from build123d import *

# Parameters (mm, degrees)
F0_R         = 1.745
F1_DEPTH     = 1.66
F2_R         = 4
F3_T1_DEPTH  = 11.0406372139
F3_T3_DEPTH  = 2.9562992506
F3_T5_DEPTH  = 2.7192996153
F3_T7_DEPTH  = 12.9650408158
F3_T9_DEPTH  = 2.8625815694
F3_T11_DEPTH = 2.7133982533


# Not quite as in the source:
# - a fillet or chamfer that OpenCascade refuses, or shapes differently, is made with other operations: its cross-section is extruded or revolved along the edge and cut away or added


with BuildPart() as f1:
    # F0 (on Top) → F1 (new body)
    with BuildSketch(Plane.XY):
        with BuildLine():
            Line((9.301183783, 21.0652845629), (-9.82, 21.0652845629))
            Line((-9.82, 21.0652845629), (-9.82, 16.2710778286))
            Line((-9.82, 16.2710778286), (-6.76, 13.7425599752))
            Line((-6.76, 13.7425599752), (-6.76, 6.5925599752))
            Line((-6.76, 6.5925599752), (-9.82, 4.2610778286))
            Line((-9.82, 4.2610778286), (-9.82, 0.8810778286))
            Line((-9.82, 0.8810778286), (-9.82, -30.8189221714))
            Line((-9.82, -30.8189221714), (-6.5227223381, -36.7505173139))
            Line((-6.5227223381, -36.7505173139), (-3.43, -30.6931023543))
            Line((-3.43, -30.6931023543), (-3.43, 0))
            ThreePointArc((-3.43, 0), (0, 3.43), (3.43, 0))
            Line((3.43, 0), (3.43, -30.6931023543))
            Line((3.43, -30.6931023543), (6.4156440855, -37.4231023543))
            Line((6.4156440855, -37.4231023543), (9.301183783, -30.87889562))
            Line((9.301183783, -30.87889562), (9.301183783, 1.0068976457))
            Line((9.301183783, 1.0068976457), (9.4504277734, 4.2610778286))
            Line((9.4504277734, 4.2610778286), (6.5356440855, 6.7183797924))
            Line((6.5356440855, 6.7183797924), (6.5356440855, 13.8683797924))
            Line((6.5356440855, 13.8683797924), (9.2185314492, 16.0852845629))
            Line((9.2185314492, 16.0852845629), (9.301183783, 21.0652845629))
        make_face()
        with Locations((-6.686183783, 18.82610438)):
            Circle(F0_R, mode=Mode.SUBTRACT)
        with Locations((6.686183783, 18.7002845629)):
            Circle(F0_R, mode=Mode.SUBTRACT)
    extrude(amount=F1_DEPTH)

    # F2
    f2_edges = [f1.edges().sort_by_distance(p)[0] for p in [
        (-6.76, 6.59256, 0.83),
        (-6.76, 13.74256, 0.83),
        (6.535644, 6.71838, 0.83),
        (6.535644, 13.86838, 0.83),
    ]]
    fillet(f2_edges, radius=F2_R)

    # F3: fillet of radius 1 on 6 edges, made by hand

    # F3_s2 → F3_t1 (cut)
    with BuildSketch(Plane.XY.offset(-4.690318607)):
        with BuildLine():
            add(Edge.make_bspline(
                [(-7.4342616517, -35.110715417), (-6.5227223381, -36.7505173139), (-5.6695955837, -35.0795807734)],
                knots=[0, 0, 0, 1, 1, 1], degree=2, weights=[1, 1, 1]))
            Line((-5.6695955837, -35.0795807734), (-6.5227223381, -36.7505173139))
            Line((-6.5227223381, -36.7505173139), (-7.4342616517, -35.110715417))
        make_face()
    extrude(amount=F3_T1_DEPTH, mode=Mode.SUBTRACT)

    # F3_s4 → F3_t3 (cut)
    with BuildSketch(Plane.XY.offset(-0.6481496253)):
        with BuildLine():
            add(Edge.make_bspline(
                [(-9.82, -30.5596623213), (-9.82, -30.8189221714), (-9.6940354517, -31.0455244716)],
                knots=[0, 0, 0, 1, 1, 1], degree=2, weights=[1, 1, 1]))
            Line((-9.6940354517, -31.0455244716), (-9.82, -30.8189221714))
            Line((-9.82, -30.8189221714), (-9.82, -30.5596623213))
        make_face()
    extrude(amount=F3_T3_DEPTH, mode=Mode.SUBTRACT)

    # F3_s6 → F3_t5 (cut)
    with BuildSketch(Plane.XY.offset(-0.5296498077)):
        with BuildLine():
            add(Edge.make_bspline(
                [(3.43, -30.4812424312), (3.43, -30.6931023543), (3.5159130776, -30.8867607393)],
                knots=[0, 0, 0, 1, 1, 1], degree=2, weights=[1, 1, 1]))
            Line((3.5159130776, -30.8867607393), (3.43, -30.6931023543))
            Line((3.43, -30.6931023543), (3.43, -30.4812424312))
        make_face()
    extrude(amount=F3_T5_DEPTH, mode=Mode.SUBTRACT)

    # F3_s8 → F3_t7 (cut)
    with BuildSketch(Plane.XY.offset(-5.6525204079)):
        with BuildLine():
            add(Edge.make_bspline(
                [(5.4987638806, -35.3563443608), (6.4156440855, -37.4231023543), (7.3278517341, -35.3542777798)],
                knots=[0, 0, 0, 1, 1, 1], degree=2, weights=[1, 1, 1]))
            Line((7.3278517341, -35.3542777798), (6.4156440855, -37.4231023543))
            Line((6.4156440855, -37.4231023543), (5.4987638806, -35.3563443608))
        make_face()
    extrude(amount=F3_T7_DEPTH, mode=Mode.SUBTRACT)

    # F3_s10 → F3_t9 (cut)
    with BuildSketch(Plane.XY.offset(-0.6012907847)):
        with BuildLine():
            add(Edge.make_bspline(
                [(-3.5393693837, -30.9073135471), (-3.43, -30.6931023543), (-3.43, -30.4525860404)],
                knots=[0, 0, 0, 1, 1, 1], degree=2, weights=[1, 1, 1]))
            Line((-3.43, -30.4525860404), (-3.43, -30.6931023543))
            Line((-3.43, -30.6931023543), (-3.5393693837, -30.9073135471))
        make_face()
    extrude(amount=F3_T9_DEPTH, mode=Mode.SUBTRACT)

    # F3_s12 → F3_t11 (cut)
    with BuildSketch(Plane.XY.offset(-0.5266991266)):
        with BuildLine():
            add(Edge.make_bspline(
                [(9.301183783, -30.6682159693), (9.301183783, -30.87889562), (9.2161847141, -31.0716676965)],
                knots=[0, 0, 0, 1, 1, 1], degree=2, weights=[1, 1, 1]))
            Line((9.2161847141, -31.0716676965), (9.301183783, -30.87889562))
            Line((9.301183783, -30.87889562), (9.301183783, -30.6682159693))
        make_face()
    extrude(amount=F3_T11_DEPTH, mode=Mode.SUBTRACT)


solid = f1.part
Could you check a few things on this model? Use its own coordinates, in mm. A direction names the side the tool comes from. Round coordinates to 2 decimals unless told otherwise and drop trailing zeros. Order: outer loops, then holes, each group sorted by start corner. A loop starts at its lowest first (then second) coordinate and runs counter-clockwise, first axis right, second up.
(1) Imagine slicing it at C-C (x = 0). Write out the boundary of the cut face in (y, z).
Response values:
outline: (3.43, 0) - (21.07, 0) - (21.07, 1.66) - (3.43, 1.66) - close
(2) Imagine slicing it at D-D (y = 7). Write out the boundary of the cut face in (x, z).
Response values:
outline: (-7.08, 0) - (6.86, 0) - (6.86, 1.66) - (-7.08, 1.66) - close
(3) Which directions (+Z, -Z, +X, -X, +Y, -Y) give clear straight access to the entire face, cutting with the end or side of a thin tool? Please do faces 1 (the flat face through (-3.43, -15, 1)), 2 (the cylindrical face through (6.9, 6.91, 0.84)), 3 (the flat face through (9.375, 2.611, 0.818)), 4 (the cylindrical face through (-7.152, 13.585, 0.842)).
Response values:
face 1: +Z, -Z, -Y
face 2: +Z, -Z, +X
face 3: +Z, -Z, +X, -Y
face 4: +Z, -Z, -X
(4) If we mould it in two halves opening along X, with no side actions, what happens to faces 5 (the cylindrical face through (6.927, 13.711, 0.842)), 6 (the cylindrical face through (-7.164, 6.821, 0.842)), 7 (the cylindrical face through (-0.08, 3.43, 0.82))? For each: released by +X, released by -X, zero draft, split by the parting line, or undercut.
Response values:
face 5: released by +X
face 6: released by -X
face 7: undercut
(5) Imagine slicing it at A-A (y = -1). Write out the boundary of the cut face in (x, z), plus the area to 3 significant figures.
Response values:
outline: (-9.82, 0) - (-3.43, 0) - (-3.43, 1.66) - (-9.82, 1.66) - close; (3.43, 0) - (9.3, 0) - (9.3, 1.66) - (3.43, 1.66) - close
area: 20.4 mm2
(6) I'm going to push flat-ended pins straight in: pin 1 (0.8 mm diameter, centred on y = 10.5, z = 0.5, fed in from +X); pin 2 (2 mm diameter, centred on x = 6.69, y = 18.7, fed in from -Z) (3 decimals). Where does each tip first touch, or does it pass through?
Response values:
pin 1: stops at x = 6.54
pin 2: passes through
(7) Imagine slicing it at B-B (z = 0.6). Count the separate pieces of the cut face and the enclosed holes in it, plus the area to 3 significant figures.
Response values:
separate pieces: 1
enclosed holes: 2
area: 727 mm2
(8) Please list where these lines run through material, in increasing order: line 1 along Y through (x, z) = (7.75, 1.2); line 2 along X through (y, z) = (-28.5, 0.95); line 3 along Y through (x, z) = (-7.75, 1.25).
Response values:
line 1: y = -34.4 to 5.71, 14.86 to 17.32, 20.08 to 21.07
line 2: x = -9.82 to -3.43, 3.43 to 9.3
line 3: y = -34.54 to 5.94, 14.49 to 17.44, 20.21 to 21.07
